```python
from build123d import *

# Parameters (mm, degrees)
SKETCH1_W                       = 150
SKETCH1_H                       = 150
BOSS_EXTRUDE1_DEPTH             = 30
FILLET1_R                       = 1
SKETCH2_R                       = 39.25
CUT_EXTRUDE4_DEPTH              = 10
TAP_DRILL_FOR_M3X0_5_TAP3_D     = 2.5
TAP_DRILL_FOR_M3X0_5_TAP3_DEPTH = 10
TAP_DRILL_FOR_M3X0_5_TAP3_TIP   = 0.751075774


with BuildPart() as part:
    # Sketch1 → Boss-Extrude1 (new body)
    with BuildSketch(Plane.XY):
        Rectangle(SKETCH1_W, SKETCH1_H)
    extrude(amount=-BOSS_EXTRUDE1_DEPTH)

    # Fillet1
    fillet1_edges = [part.edges().sort_by_distance(p)[0] for p in [
        (0, 75, -30),
        (-75, 0, 0),
        (0, 75, 0),
        (75, 0, 0),
        (0, -75, 0),
        (-75, -75, -15),
        (-75, 75, -15),
        (75, 75, -15),
        (75, -75, -15),
        (75, 0, -30),
    ]]
    fillet(fillet1_edges, radius=FILLET1_R)

    # Sketch2 → Cut-Extrude4 (cut)
    with BuildSketch(Plane.XY):
        Circle(SKETCH2_R)
    extrude(amount=-CUT_EXTRUDE4_DEPTH, mode=Mode.SUBTRACT)

    # Tap Drill for M3x0.5 Tap3
    with Locations(Plane.XY):
        with Locations((0.496213053, 46.5), (-48.237547134, -16.547252974)):
            Hole(TAP_DRILL_FOR_M3X0_5_TAP3_D / 2, depth=TAP_DRILL_FOR_M3X0_5_TAP3_DEPTH)
            with Locations((0, 0, -(TAP_DRILL_FOR_M3X0_5_TAP3_DEPTH + TAP_DRILL_FOR_M3X0_5_TAP3_TIP / 2))):  # 118° drill point
                Cone(0, TAP_DRILL_FOR_M3X0_5_TAP3_D / 2, TAP_DRILL_FOR_M3X0_5_TAP3_TIP, mode=Mode.SUBTRACT)


solid = part.part
```
Model file for the job. Use its own axes, mm. A direction names the side the tool comes from. Coordinates: 2 decimals unless noted, no trailing zeros. Loops run counter-clockwise (first coordinate to the right, second up) from the corner with the lowest first, then second, coordinate; pieces in that order, holes last. Notation, with made-up numbers: M -1,61 L 31,61 A15 ccw 31,86 Z; hole C 83.5,-6 d6. An arc over 180 degrees is marked long. Use CSV: the item, a comma, the result in double quotes. Start each with the question number.
1. Flat gauge pins, fed straight in: pin 1 (4 mm diameter, centred on x = 3, y = -4, fed in from +Z); pin 2 (1.5 mm diameter, centred on x = -48.24, y = -16.55, fed in from +Z). Where does each tip first touch, or does it go through?
2. Band-saw the part on C-C, the plane x = 36.5. List the corners of the cut face in (y, z), then the cut area to 3 significant figures.
3. Two-plate mould, pull along X, no slides. Class faces 3 (the flat face through (-1, 75, -15)), 4 (the flat face through (-75, -1, -15)), 5 (the cylindrical face through (-39.21, 1.73, -4.93)): pulls with the +X half, pulls with the -X half, needs draft (parallel to the pull), parting line crosses it, or undercut.
4. Band-saw the part on B-B, the plane z = -7.25. List the corners of the cut face in (x, y), then the cut area to 3 significant figures.
5. Band-saw the part on A-A, the plane y = 0. List the corners of the cut face in (x, z), then the cut area to 3 significant figures.
6. Tool access for faces 1 (the flat face through (-1, 1, -10)), 2 (the flat face through (-34, 34, 0)): list every direction of +Z, -Z, +X, -X, +Y, -Y with a clear straight run to the whole face (end or side of a thin tool).
7. Probe probe 1 along X at (y, z) = (46.5, -3.25); probe 2 along Z at (x, y) = (22, -31); probe 3 along Y at (x, z) = (9, -4.75). List the from-to ranges inside material, lowest first. Write a range as [from, to].
Entries:
1,pin 1,"stops at z = -10"
1,pin 2,"stops at z = -10.3"
2,outline,"M -75,-30 L 74,-30 A1 ccw 75,-29 L 75,-1 A1 ccw 74,0 L 14.43,0 L 14.43,-10 L -14.43,-10 L -14.43,0 L -74,0 A1 ccw -75,-1 Z"
2,area,"4,210 mm2"
3,face 3,"needs draft"
3,face 4,"pulls with the -X half"
3,face 5,"undercut"
4,outline,"M -75,-74 A1 ccw -74,-75 L 74,-75 A1 ccw 75,-74 L 75,74 A1 ccw 74,75 L -74,75 A1 ccw -75,74 Z; hole C -48.24,-16.55 d2.5; hole C 0,0 d78.5; hole C 0.5,46.5 d2.5"
4,area,"17,600 mm2"
5,outline,"M -75,-30 L 74,-30 A1 ccw 75,-29 L 75,-1 A1 ccw 74,0 L 39.25,0 L 39.25,-10 L -39.25,-10 L -39.25,0 L -74,0 A1 ccw -75,-1 Z"
5,area,"3,710 mm2"
6,face 1,"+Z"
6,face 2,"+Z, +X, -X, +Y, -Y"
7,probe 1,"x = [-75, -0.75], [1.75, 75]"
7,probe 2,"z = [-30, -10]"
7,probe 3,"y = [-75, -38.2], [38.2, 75]"
